The figure shows three views and two pictorial views of one solid part (mm, origin at its lowest corner). Answer the questions. A direction names the side the tool comes from. Round coordinates to 2 decimals unless told otherwise and drop trailing zeros. Loops run counter-clockwise (first coordinate to the right, second up) from the corner with the lowest first, then second, coordinate; pieces in that order, holes last. Notation, with made-up numbers: (-38, 33) -> (20, 33) arc R16 ccw to (20, 37) -> close; hole circle Ø3 at (50, 70). An arc over 180 degrees is marked (long way). Write item = value, one per line. Start each with the question number.
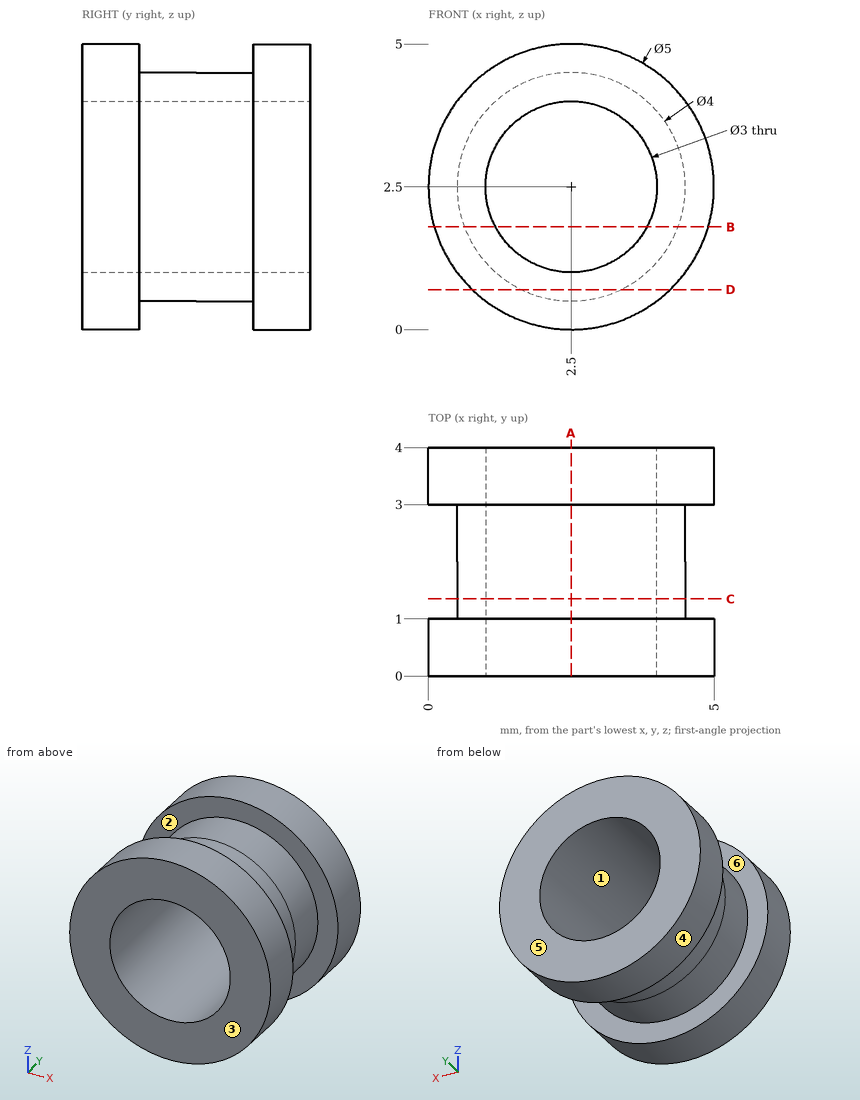
Item 1: Section D-D (z = 0.7) is taken. Determine the outline of the cut face in (x, y).
Item 2: A flat-ended cylindrical pin translates along its axis: pin 1 (1 mm diameter, centred on y = 3, z = 1.5, fed in from -X). Find the tip coordinate at first contact, or state that the pin passes through.
Item 3: A tool of negligible diameter and unlimited length cuts with its end or side. For the marked faces 1 and 2, from which of +Z, -Z, +X, -X, +Y, -Y can it reach the whole face along a straight path? Write none if from no direction.
Item 4: Find the intervals of material crossed by line 1 along Z through (x, y) = (2.5, 2.4); line 2 along Y through (x, z) = (4.65, 3.15); line 3 along Z through (x, y) = (3.05, 3.05), in increasing order. Write a range as [from, to].
Item 5: The mould has two halves that part along Y. Classify the marked faces 3, 4, 5 and 6: pulls with the +Y half, pulls with the -Y half, needs draft (parallel to the pull), parting line crosses it, or undercut.
Item 6: Section C-C (y = 1.35) is taken. Determine the outline of the cut face in (x, z), then the cut area to 3 significant figures.
Item 7: Section A-A (x = 2.5) is taken. Determine the outline of the cut face in (y, z), then the cut area to 3 significant figures.
Item 8: Section B-B (z = 1.8) is taken. Determine the outline of the cut face in (x, y), then the cut area to 3 significant figures.
Worked answers:
q1.outline = (0.77, 0) -> (4.23, 0) -> (4.23, 1) -> (3.37, 1) -> (3.37, 3) -> (4.23, 3) -> (4.23, 4) -> (0.77, 4) -> (0.77, 3) -> (1.63, 3) -> (1.63, 1) -> (0.77, 1) -> close
q2.pin_1 = 0.05
q3.face_1 = +Y, -Y
q3.face_2 = none
q4.line_1 = [0.5, 1], [4, 4.5]
q4.line_2 = [0, 1], [3, 4]
q4.line_3 = [0.06, 1.1], [3.9, 4.94]
q5.face_3 = pulls with the -Y half
q5.face_4 = needs draft
q5.face_5 = pulls with the +Y half
q5.face_6 = undercut
q6.outline = circle Ø4 at (2.5, 2.5); hole circle Ø3 at (2.5, 2.5)
q6.area = 5.50 mm2
q7.outline = (0, 0) -> (1, 0) -> (1, 0.5) -> (3, 0.5) -> (3, 0) -> (4, 0) -> (4, 1) -> (0, 1) -> close; (0, 4) -> (4, 4) -> (4, 5) -> (3, 5) -> (3, 4.5) -> (1, 4.5) -> (1, 5) -> (0, 5) -> close
q7.area = 6.00 mm2
q8.outline = (0.1, 0) -> (1.17, 0) -> (1.17, 4) -> (0.1, 4) -> (0.1, 3) -> (0.63, 3) -> (0.63, 1) -> (0.1, 1) -> close; (3.83, 0) -> (4.9, 0) -> (4.9, 1) -> (4.37, 1) -> (4.37, 3) -> (4.9, 3) -> (4.9, 4) -> (3.83, 4) -> close
q8.area = 6.48 mm2
